Print and shaded views of the part. All mm, measured from the part's lowest x, y and z. Give positions to 0.01 mm unless a question says otherwise; leave off trailing zeros. Answer as a JSON object with one key per item and string values. Group by question number.
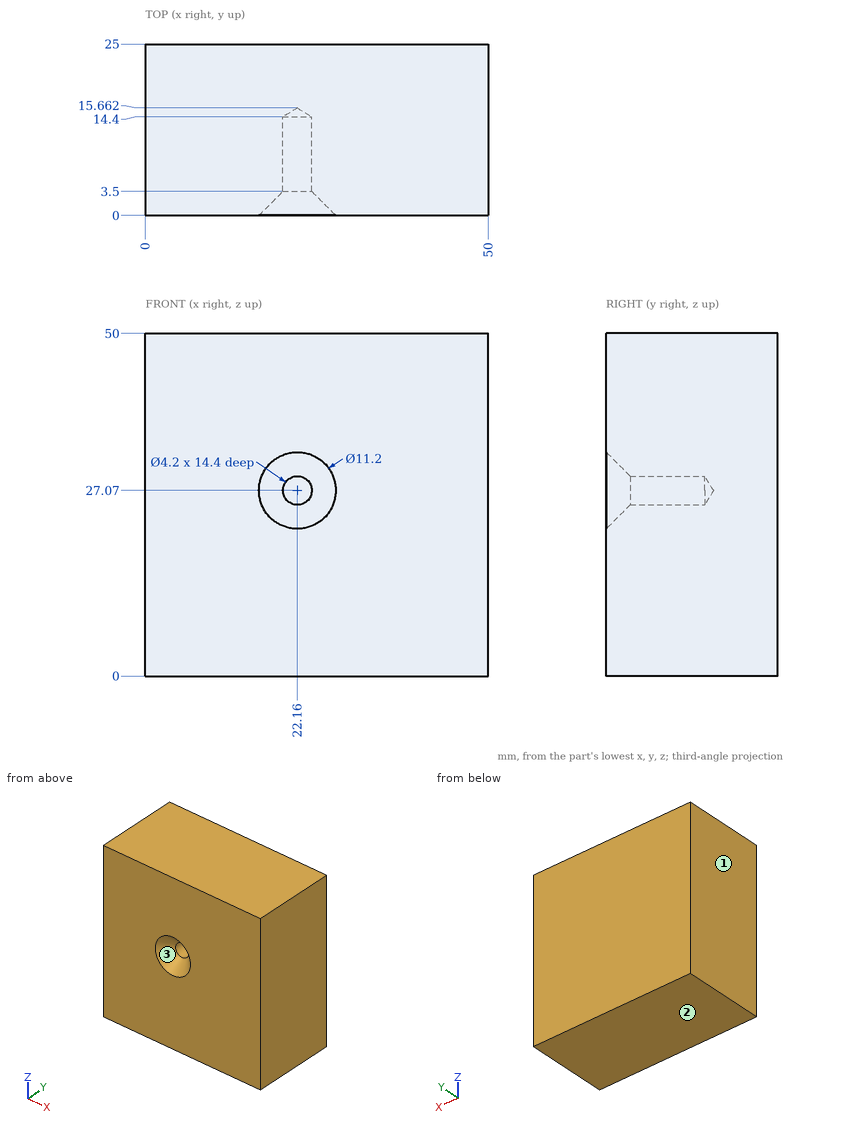
(1) Probe line 1 along X through (y, z) = (13, 26) (1 decimal); line 2 along Y through (x, z) = (25.5, 23.5). List the from-to ranges inside material, lowest first. Write a range as [from, to].
(2) Pull direction X, two halves, no side cores. Call the marked faces 1, 2 and 3: pulls with the +X half, pulls with the -X half, needs draft (parallel to the pull), parting line crosses it, or undercut.
(3) Pin check, flat tip, straight feed: pin 1 (6 mm diameter, centred on x = 20.5, z = 8.5, fed in from -Y). Stop position of the tip, or through.
Calculated:
{
 "1": {"line 1": "x = [0, 20.4], [24, 50]", "line 2": "y = [0.71, 25]"},
 "2": {"face 1": "pulls with the -X half", "face 2": "needs draft", "face 3": "undercut"},
 "3": {"pin 1": "stops at y = 0"}
}
